Input: dimensioned drawing with shaded views. Units: mm. Origin: part minimum x, y, z. Give positions to 0.01 mm unless a question says otherwise; leave off trailing zeros. Write each loop counter-clockwise with the first axis right and the second up, starting at its lowest first coordinate (ties: lowest second). Pieces come first, ordered by that corner, then holes. Notation, with made-up numbers: (43.25, -23.75) -> (89.25, -23.75) arc R18 ccw to (89.25, -19.75) -> close; hole circle Ø8 at (-29.75, -32.75). An arc over 180 degrees is marked (long way). Answer as a JSON object with one key per item and string values.
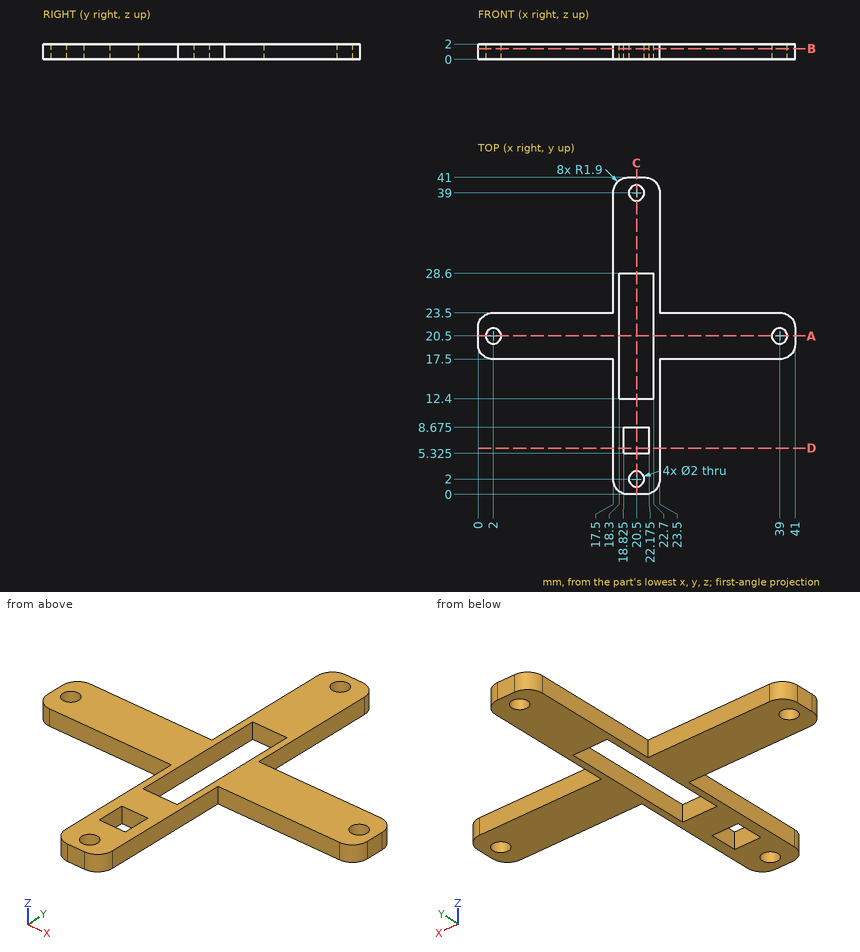
Q1. Cut plane D-D (y = 6). Return the cut outline in (x, z) (3 decimals).
Values:
{"outline": "(17.5, 0) -> (18.825, 0) -> (18.825, 2) -> (17.5, 2) -> close; (22.175, 0) -> (23.5, 0) -> (23.5, 2) -> (22.175, 2) -> close"}
Q2. Material intervals for L1, parallel to Y at x = 20.5, z = 1.55 (3 decimals); L2, parallel to X at y = 17, z = 1; L3, parallel to Y at x = 2, z = 0.95, sorted ascending. Write a range as from..to.
Values:
{"L1": "0..1, 3..5.325, 8.675..12.4, 28.6..38, 40..41", "L2": "17.5..18.3, 22.7..23.5", "L3": "17.5..19.5, 21.5..23.5"}
Q3. Cut plane C-C (x = 20.5). Return the cut outline in (y, z) (3 decimals).
Values:
{"outline": "(0, 0) -> (1, 0) -> (1, 2) -> (0, 2) -> close; (3, 0) -> (5.325, 0) -> (5.325, 2) -> (3, 2) -> close; (8.675, 0) -> (12.4, 0) -> (12.4, 2) -> (8.675, 2) -> close; (28.6, 0) -> (38, 0) -> (38, 2) -> (28.6, 2) -> close; (40, 0) -> (41, 0) -> (41, 2) -> (40, 2) -> close"}
Q4. Cut plane B-B (z = 1.4). State how many separate pieces and enclosed holes the cut face has, and give its area (3 significant figures).
Values:
{"separate pieces": "1", "enclosed holes": "6", "area": "355 mm²"}
Q5. First-contact query: P1, Ø1, axis at y = 10, z = 1, coming from the -X side; P2, Ø0.6, axis at y = 34, z = 1, coming from the +X side; P3, Ø0.6, axis at x = 9, z = 1.5, coming from the -Y side; P4, Ø6, axis at x = 31, y = 27.5, coming from the +Z side. Flat tips, straight axial feed; report the tip coordinate or a pass-through.
Values:
{"P1": "x = 17.5", "P2": "x = 23.5", "P3": "y = 17.5", "P4": "through"}
Q6. Cut plane A-A (y = 20.5). Return the cut outline in (x, z), and give its area (3 significant figures).
Values:
{"outline": "(0, 0) -> (1, 0) -> (1, 2) -> (0, 2) -> close; (3, 0) -> (18.3, 0) -> (18.3, 2) -> (3, 2) -> close; (22.7, 0) -> (38, 0) -> (38, 2) -> (22.7, 2) -> close; (40, 0) -> (41, 0) -> (41, 2) -> (40, 2) -> close", "area": "65.2 mm²"}
